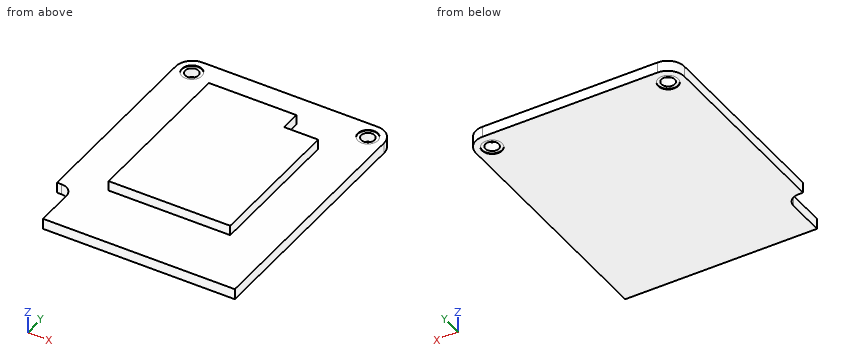
```python
from build123d import *

# Parameters (mm, degrees)
SKETCH1_R           = 1.5
BOSS_EXTRUDE1_DEPTH = 1.6
BOSS_EXTRUDE2_START = 0.1
SKETCH1_5_R         = 1.5
SKETCH1_5_R_2       = 1
BOSS_EXTRUDE2_DEPTH = 1.4
BOSS_EXTRUDE3_DEPTH = 1.5


with BuildPart() as part:
    # Sketch1 → Boss-Extrude1 (new body)
    with BuildSketch(Plane.XY):
        with BuildLine():
            Line((-15.6, 17), (-15.6, -12))
            Line((-15.6, -12), (-14.9, -12))
            ThreePointArc((-14.9, -12), (-13.627207794, -12.527207794), (-13.1, -13.8))
            Line((-13.1, -13.8), (-13.1, -19.5))
            Line((-13.1, -19.5), (15.6, -19.5))
            Line((15.6, -19.5), (15.6, 17))
            ThreePointArc((15.6, 17), (14.867766953, 18.767766953), (13.1, 19.5))
            Line((13.1, 19.5), (-13.1, 19.5))
            ThreePointArc((-13.1, 19.5), (-14.867766953, 18.767766953), (-15.6, 17))
        make_face()
        with Locations((-13.17, 17)):
            Circle(SKETCH1_R, mode=Mode.SUBTRACT)
        with Locations((13.17, 17)):
            Circle(SKETCH1_R, mode=Mode.SUBTRACT)
    extrude(amount=BOSS_EXTRUDE1_DEPTH)

    # Sketch1<5> → Boss-Extrude2 (add)
    with BuildSketch(Plane.XY.offset(BOSS_EXTRUDE2_START)):
        with Locations((13.17, 17)):
            Circle(SKETCH1_5_R)
        with Locations((13.17, 17)):
            Circle(SKETCH1_5_R_2, mode=Mode.SUBTRACT)
        with Locations((-13.17, 17)):
            Circle(SKETCH1_5_R)
        with Locations((-13.17, 17)):
            Circle(SKETCH1_5_R_2, mode=Mode.SUBTRACT)
    extrude(amount=BOSS_EXTRUDE2_DEPTH)

    # Sketch2 → Boss-Extrude3 (add)
    with BuildSketch(Plane.XY.offset(1.6)):
        Polygon((-9.1, 14.5), (4, 14.5), (4, 11.5), (9.1, 11.5), (9.1, -10), (-9.1, -10), align=None)
    extrude(amount=BOSS_EXTRUDE3_DEPTH)


solid = part.part
```
Design review of the part built by this model. Coordinates are the model's own, in mm. Coordinates: 2 decimals unless noted, no trailing zeros. Loops run counter-clockwise (first coordinate to the right, second up) from the corner with the lowest first, then second, coordinate; pieces in that order, holes last. Notation, with made-up numbers: (-21, -13) -> (18, -13) arc R22 cw to (18, -7) -> close; hole circle Ø10 at (12.5, 74). An arc over 180 degrees is marked (long way). Answer as a JSON object with one key per item and string values.
Q1. Take a section at A-A on y = 13. Give the boundary of the cut face in (x, z).
Answer block:
{"outline": "(-15.6, 0) -> (15.6, 0) -> (15.6, 1.6) -> (4, 1.6) -> (4, 3.1) -> (-9.1, 3.1) -> (-9.1, 1.6) -> (-15.6, 1.6) -> close"}
Q2. Clearance check with flat-ended pins moving along their axes: pin 1 Ø1.3 at (y, z) = (-17, 1) entering from -X; pin 2 Ø2.5 at (x, y) = (-13.17, 17) entering from +Z; pin 3 Ø3.5 at (x, y) = (13, 16.5) entering from +Z; pin 4 Ø1.8 at (x, y) = (-13.17, 17) entering from +Z. State where each tip first meets the part, or that it passes through.
Answer block:
{"pin 1": "stops at x = -13.1", "pin 2": "stops at z = 1.5", "pin 3": "stops at z = 1.6", "pin 4": "passes through"}
Q3. To check wall thickness, follow L1, parallel to Y at x = 13.17, z = 1.55; L2, parallel to Z at x = -12.5, y = -14; L3, parallel to Y at x = 1, z = 2.95. State the ranges of each line that lie inside material, in increasing order.
Answer block:
{"L1": "y = -19.5 to 15.5, 18.5 to 19.5", "L2": "z = 0 to 1.6", "L3": "y = -10 to 14.5"}
Q4. Take a section at B-B on z = 0.55. Give the boundary of the cut face in (x, y).
Answer block:
{"outline": "(-15.6, -12) -> (-14.9, -12) arc R1.8 cw to (-13.1, -13.8) -> (-13.1, -19.5) -> (15.6, -19.5) -> (15.6, 17) arc R2.5 ccw to (13.1, 19.5) -> (-13.1, 19.5) arc R2.5 ccw to (-15.6, 17) -> close; hole circle Ø2 at (-13.17, 17); hole circle Ø2 at (13.17, 17)"}
Q5. Take a section at C-C on x = 11. Give the boundary of the cut face in (y, z), plus the area to 3 significant figures.
Answer block:
{"outline": "(-19.5, 0) -> (19.5, 0) -> (19.5, 1.6) -> (-19.5, 1.6) -> close", "area": "62.4 mm^2"}
Q6. Take a section at D-D on y = -11.5. Give the boundary of the cut face in (x, z), plus the area to 3 significant figures.
Answer block:
{"outline": "(-15.6, 0) -> (15.6, 0) -> (15.6, 1.6) -> (-15.6, 1.6) -> close", "area": "49.9 mm^2"}
